from build123d import *

# Parameters (mm, degrees)
BOSS_EXTRUDE1_DEPTH = 70
CUT_EXTRUDE1_REACH  = 72
SKETCH14_R          = 4
CUT_EXTRUDE2_REACH  = 19
SKETCH15_R          = 3.25
CUT_EXTRUDE3_REACH  = 72
SKETCH16_W          = 57.95105002
SKETCH16_H          = 16.678137539
SKETCH17_R          = 19.15
CUT_EXTRUDE4_DEPTH  = 2
CUT_EXTRUDE5_REACH  = 7.672
SKETCH18_R          = 10
CUT_EXTRUDE6_REACH  = 9.672
SKETCH19_R          = 2.5
SKETCH19_R_2        = 2.7
SKETCH19_R_3        = 2.618497629


with BuildPart() as part:
    # Sketch12 → Boss-Extrude1 (new body)
    with BuildSketch(Plane(origin=(0, 0, 0), x_dir=(0, 0, -1), z_dir=(1, 0, 0))):
        Polygon((70.005446089, -2.999997853), (-70, -2.999997853), (-70, 14.000002147), (-50, 14.000002147), (-50, 20.000002147), (50, 20.000002147), (50, 14.000002147), (70.005446089, 14.000002147), align=None)
    extrude(amount=BOSS_EXTRUDE1_DEPTH)

    # Sketch14 → Cut-Extrude1 (cut, up to next)
    with BuildSketch(Plane.ZY, mode=Mode.PRIVATE) as cut_extrude1_sk1:
        with Locations((-40, 10.000001073)):
            Circle(SKETCH14_R)
    cut_extrude1_tool1 = extrude(cut_extrude1_sk1.sketch, amount=-CUT_EXTRUDE1_REACH, mode=Mode.PRIVATE) & part.part
    add(cut_extrude1_tool1.solids().sort_by_distance((0, 10.000001, -40))[0], mode=Mode.SUBTRACT)
    # Sketch14 → Cut-Extrude1 (cut, up to next)
    with BuildSketch(Plane.ZY, mode=Mode.PRIVATE) as cut_extrude1_sk2:
        with Locations((40, 10.000001073)):
            Circle(SKETCH14_R)
    cut_extrude1_tool2 = extrude(cut_extrude1_sk2.sketch, amount=-CUT_EXTRUDE1_REACH, mode=Mode.PRIVATE) & part.part
    add(cut_extrude1_tool2.solids().sort_by_distance((0, 10.000001, 40))[0], mode=Mode.SUBTRACT)

    # Sketch15 → Cut-Extrude2 (cut, up to next)
    with BuildSketch(Plane(origin=(0, 14.000002147, 0), x_dir=(1, 0, 0), z_dir=(0, 1, 0)), mode=Mode.PRIVATE) as cut_extrude2_sk1:
        with Locations((50, 60.002723044)):
            Circle(SKETCH15_R)
    cut_extrude2_tool1 = extrude(cut_extrude2_sk1.sketch, amount=-CUT_EXTRUDE2_REACH, mode=Mode.PRIVATE) & part.part
    add(cut_extrude2_tool1.solids().sort_by_distance((50, 14.000002, -60.002723))[0], mode=Mode.SUBTRACT)
    # Sketch15 → Cut-Extrude2 (cut, up to next)
    with BuildSketch(Plane(origin=(0, 14.000002147, 0), x_dir=(1, 0, 0), z_dir=(0, 1, 0)), mode=Mode.PRIVATE) as cut_extrude2_sk2:
        with Locations((20, 60.002723044)):
            Circle(SKETCH15_R)
    cut_extrude2_tool2 = extrude(cut_extrude2_sk2.sketch, amount=-CUT_EXTRUDE2_REACH, mode=Mode.PRIVATE) & part.part
    add(cut_extrude2_tool2.solids().sort_by_distance((20, 14.000002, -60.002723))[0], mode=Mode.SUBTRACT)
    # Sketch15 → Cut-Extrude2 (cut, up to next)
    with BuildSketch(Plane(origin=(0, 14.000002147, 0), x_dir=(1, 0, 0), z_dir=(0, 1, 0)), mode=Mode.PRIVATE) as cut_extrude2_sk3:
        with Locations((50, -60)):
            Circle(SKETCH15_R)
    cut_extrude2_tool3 = extrude(cut_extrude2_sk3.sketch, amount=-CUT_EXTRUDE2_REACH, mode=Mode.PRIVATE) & part.part
    add(cut_extrude2_tool3.solids().sort_by_distance((50, 14.000002, 60))[0], mode=Mode.SUBTRACT)
    # Sketch15 → Cut-Extrude2 (cut, up to next)
    with BuildSketch(Plane(origin=(0, 14.000002147, 0), x_dir=(1, 0, 0), z_dir=(0, 1, 0)), mode=Mode.PRIVATE) as cut_extrude2_sk4:
        with Locations((20, -60)):
            Circle(SKETCH15_R)
    cut_extrude2_tool4 = extrude(cut_extrude2_sk4.sketch, amount=-CUT_EXTRUDE2_REACH, mode=Mode.PRIVATE) & part.part
    add(cut_extrude2_tool4.solids().sort_by_distance((20, 14.000002, 60))[0], mode=Mode.SUBTRACT)

    # Sketch16 → Cut-Extrude3 (cut, up to next)
    with BuildSketch(Plane.ZY, mode=Mode.PRIVATE) as cut_extrude3_sk1:
        with Locations((0, 13.011297134)):
            Rectangle(SKETCH16_W, SKETCH16_H)
    cut_extrude3_tool1 = extrude(cut_extrude3_sk1.sketch, amount=-CUT_EXTRUDE3_REACH, mode=Mode.PRIVATE) & part.part
    add(cut_extrude3_tool1.solids().sort_by_distance((0, 13.011297, 0))[0], mode=Mode.SUBTRACT)

    # Sketch17 → Cut-Extrude4 (cut)
    with BuildSketch(Plane(origin=(0, 4.672228364, 0), x_dir=(1, 0, 0), z_dir=(0, 1, 0))):
        with Locations((35, 0)):
            Circle(SKETCH17_R)
    extrude(amount=-CUT_EXTRUDE4_DEPTH, mode=Mode.SUBTRACT)

    # Sketch18 → Cut-Extrude5 (cut, up to next)
    with BuildSketch(Plane(origin=(0, 2.672228364, 0), x_dir=(1, 0, 0), z_dir=(0, 1, 0)), mode=Mode.PRIVATE) as cut_extrude5_sk1:
        with Locations((35, 0)):
            Circle(SKETCH18_R)
    cut_extrude5_tool1 = extrude(cut_extrude5_sk1.sketch, amount=-CUT_EXTRUDE5_REACH, mode=Mode.PRIVATE) & part.part
    add(cut_extrude5_tool1.solids().sort_by_distance((35, 2.672228, 0))[0], mode=Mode.SUBTRACT)

    # Sketch19 → Cut-Extrude6 (cut, up to next)
    with BuildSketch(Plane(origin=(0, 4.672228364, 0), x_dir=(1, 0, 0), z_dir=(0, 1, 0)), mode=Mode.PRIVATE) as cut_extrude6_sk1:
        with Locations((11, 24)):
            Circle(SKETCH19_R)
    cut_extrude6_tool1 = extrude(cut_extrude6_sk1.sketch, amount=-CUT_EXTRUDE6_REACH, mode=Mode.PRIVATE) & part.part
    add(cut_extrude6_tool1.solids().sort_by_distance((11, 4.672228, -24))[0], mode=Mode.SUBTRACT)
    # Sketch19 → Cut-Extrude6 (cut, up to next)
    with BuildSketch(Plane(origin=(0, 4.672228364, 0), x_dir=(1, 0, 0), z_dir=(0, 1, 0)), mode=Mode.PRIVATE) as cut_extrude6_sk2:
        with Locations((59, 24)):
            Circle(SKETCH19_R_2)
    cut_extrude6_tool2 = extrude(cut_extrude6_sk2.sketch, amount=-CUT_EXTRUDE6_REACH, mode=Mode.PRIVATE) & part.part
    add(cut_extrude6_tool2.solids().sort_by_distance((59, 4.672228, -24))[0], mode=Mode.SUBTRACT)
    # Sketch19 → Cut-Extrude6 (cut, up to next)
    with BuildSketch(Plane(origin=(0, 4.672228364, 0), x_dir=(1, 0, 0), z_dir=(0, 1, 0)), mode=Mode.PRIVATE) as cut_extrude6_sk3:
        with Locations((59, -24)):
            Circle(SKETCH19_R_3)
    cut_extrude6_tool3 = extrude(cut_extrude6_sk3.sketch, amount=-CUT_EXTRUDE6_REACH, mode=Mode.PRIVATE) & part.part
    add(cut_extrude6_tool3.solids().sort_by_distance((59, 4.672228, 24))[0], mode=Mode.SUBTRACT)
    # Sketch19 → Cut-Extrude6 (cut, up to next)
    with BuildSketch(Plane(origin=(0, 4.672228364, 0), x_dir=(1, 0, 0), z_dir=(0, 1, 0)), mode=Mode.PRIVATE) as cut_extrude6_sk4:
        with Locations((11, -24)):
            Circle(SKETCH19_R_2)
    cut_extrude6_tool4 = extrude(cut_extrude6_sk4.sketch, amount=-CUT_EXTRUDE6_REACH, mode=Mode.PRIVATE) & part.part
    add(cut_extrude6_tool4.solids().sort_by_distance((11, 4.672228, 24))[0], mode=Mode.SUBTRACT)


solid = part.part
Work out the finished part from the listing and answer in its coordinate system (mm). A direction names the side the tool comes from. Give positions to 0.01 mm unless a question says otherwise; leave off trailing zeros. Loops run counter-clockwise (first coordinate to the right, second up) from the corner with the lowest first, then second, coordinate; pieces in that order, holes last. Notation, with made-up numbers: (-8, 35.5) - (25, 35.5) arc R19 ccw to (25, 46.5) - close; hole circle Ø1 at (1.5, 12). An arc over 180 degrees is marked (long way). Answer in a Markdown table with one row per item.
(1) A tool of negligible diameter and unlimited length cuts with its end or side. For faces 4 (the face through (35, 14, 60)), 5 (the face through (52.69, 3.69, 7.33)), 6 (the face through (0, 4, -1)), 7 (the face through (51.75, 5.62, -62.74)), 8 (the face through (35, 12, -28.976)), from which of +Z, -Z, +X, -X, +Y, -Y can it reach the whole face along a straight path? Write none if from no direction.
Results list:
| item | result |
|---|---|
| face 4 | +Z, +X, -X, +Y |
| face 5 | +Y |
| face 6 | +Z, -Z, -X, +Y, -Y |
| face 7 | +Y, -Y |
| face 8 | +X, -X, +Y |
(2) Consider L1, parallel to X at y = 0, z = -24; L2, parallel to Z at x = 6, y = 18.25; L3, parallel to X at y = 9.5, z = 60. Determine where each line is inside the solid, lowest interval first. Write a range as [from, to].
Results list:
| item | result |
|---|---|
| L1 | x = [0, 8.5], [13.5, 56.3], [61.7, 70] |
| L2 | z = [-50, -28.98], [28.98, 50] |
| L3 | x = [0, 16.75], [23.25, 46.75], [53.25, 70] |
(3) Section A-A (z = 0) is taken. Give the vertices of the cut face in (x, y).
Results list:
| item | result |
|---|---|
| outline | (0, -3) - (25, -3) - (25, 2.67) - (15.85, 2.67) - (15.85, 4.67) - (0, 4.67) - close; (45, -3) - (70, -3) - (70, 4.67) - (54.15, 4.67) - (54.15, 2.67) - (45, 2.67) - close |
(4) Section D-D (x = 32.5) is taken. Give the vertices of the cut face in (y, z).
Results list:
| item | result |
|---|---|
| outline | (-3, -70.01) - (14, -70.01) - (14, -50) - (20, -50) - (20, -28.98) - (4.67, -28.98) - (4.67, -18.99) - (2.67, -18.99) - (2.67, -9.68) - (-3, -9.68) - close; (-3, 9.68) - (2.67, 9.68) - (2.67, 18.99) - (4.67, 18.99) - (4.67, 28.98) - (20, 28.98) - (20, 50) - (14, 50) - (14, 70) - (-3, 70) - close; hole circle Ø8 at (10, -40); hole circle Ø8 at (10, 40) |
(5) Flat-ended cylindrical pins translate along their axes: pin 1 Ø5 at (x, z) = (50, 60) entering from +Y; pin 2 Ø6.5 at (x, y) = (29.5, 18) entering from +Z; pin 3 Ø8.5 at (x, z) = (20, -60) entering from +Y; pin 4 Ø7 at (x, z) = (59, 24) entering from +Y. Find the tip coordinate at first contact, or state that the pin passes through.
Results list:
| item | result |
|---|---|
| pin 1 | passes through |
| pin 2 | stops at z = 50 |
| pin 3 | stops at y = 14 |
| pin 4 | stops at y = 4.67 |
(6) Section C-C (z = 60) is taken. Give the vertices of the cut face in (x, y), and give its area (3 significant figures).
Results list:
| item | result |
|---|---|
| outline | (0, -3) - (16.75, -3) - (16.75, 14) - (0, 14) - close; (23.25, -3) - (46.75, -3) - (46.75, 14) - (23.25, 14) - close; (53.25, -3) - (70, -3) - (70, 14) - (53.25, 14) - close |
| area | 969 mm² |
(7) Section B-B (x = 59) is taken. Give the vertices of the cut face in (y, z), and give its area (3 significant figures).
Results list:
| item | result |
|---|---|
| outline | (-3, -70.01) - (14, -70.01) - (14, -50) - (20, -50) - (20, -28.98) - (4.67, -28.98) - (4.67, -26.7) - (-3, -26.7) - close; (-3, -21.3) - (4.67, -21.3) - (4.67, 21.38) - (-3, 21.38) - close; (-3, 26.62) - (4.67, 26.62) - (4.67, 28.98) - (20, 28.98) - (20, 50) - (14, 50) - (14, 70) - (-3, 70) - close; hole circle Ø8 at (10, -40); hole circle Ø8 at (10, 40) |
| area | 1,910 mm² |
(8) For a pull along Y with two mould halves and no side action, classify faces 1 (the face through (35, 20, -39)), 2 (the face through (35, 10, 36)), 3 (the face through (35, 17, 50)) as pulls with the +Y half, pulls with the -Y half, needs draft (parallel to the pull), parting line crosses it, or undercut.
Results list:
| item | result |
|---|---|
| face 1 | pulls with the +Y half |
| face 2 | undercut |
| face 3 | needs draft |
